Check sheet for the modelled part. Datum: model origin and axes. Units: mm. Face numbers are marked on the shaded views. A direction names the side the tool comes from. Round coordinates to 2 decimals unless told otherwise and drop trailing zeros. Write each loop counter-clockwise with the first axis right and the second up, starting at its lowest first coordinate (ties: lowest second). Pieces come first, ordered by that corner, then holes. Notation, with made-up numbers: M 50,50.5 L 67,50.5 A32 ccw 67,85.5 Z; hole C 29,73.25 d11. An arc over 180 degrees is marked long. Answer in a Markdown table with one row per item.
Autodesk Inventor part; units mm, degrees
ref_plane "YZ Plane" through (0, 0, 0) normal (1, 0, 0) x (0, 1, 0)
ref_plane "XZ Plane" through (0, 0, 0) normal (0, 1, 0) x (-1, 0, 0)
ref_plane "XY Plane" through (0, 0, 0) normal (0, 0, 1) x (1, 0, 0)
sketch "Sketch1" plane through (0, 0, 0) normal (0, 0, 1) x (1, 0, 0)
  line L0 (0, 0) -> (-122.2022, 0)
  line L1 (-122.2022, 0) -> (-122.2022, -1490)
  line L2 (-122.2022, -1490) -> (0, -1490)
  line L3 (0, -1490) -> (0, 0)
  line L4 (-122.2022, -1390) -> (-66, -1390)
  line L5 (-66, -1390) -> (-66, -1385)
  line L6 (-66, -1385) -> (-122.2022, -1385)
  line L7 (-122.2022, -1385) -> (-122.2022, -1390)
  line L8 (-122.2022, -893.3333) -> (-66, -893.3333)
  line L9 (-66, -893.3333) -> (-66, -888.3333)
  line L10 (-66, -888.3333) -> (-122.2022, -888.3333)
  line L11 (-122.2022, -888.3333) -> (-122.2022, -893.3333)
  line L12 (-122.2022, -396.6667) -> (-66, -396.6667)
  line L13 (-66, -396.6667) -> (-66, -391.6667)
  line L14 (-66, -391.6667) -> (-122.2022, -391.6667)
  line L15 (-122.2022, -391.6667) -> (-122.2022, -396.6667)
  circle A0 centre (-122.2022, -155) radius 30
  point P0 (-122.2022, -1385)
  point P1 (-122.2022, -125)
  point P2 (-122.2022, -185)
  dimension "d0" = 1490
  dimension "d1" = 122.2022
  dimension "d2" = 5
  dimension "d4" = 100
  dimension "d7" = 496.6667
  dimension "d23" = 66
  dimension "d28" = 60
  dimension "d29" = 1335
extrude "Plate1" add sketch "Sketch1" along normal blind 4 contours L3 L2 L1 L4 L5 L6 L8 L9 L10 L12 L13 L14 A0 L0
sketch "Sketch2" plane through (4, 0, 0) normal (-1, 0, 0) x (0, -1, 0)
  line L0 (1490, 0) -> (0, 0)
  line L1 (0, 0) -> (0, 60)
  line L2 (0, 60) -> (1490, 60)
  line L3 (1490, 60) -> (1490, 0)
edge flange "Flange1" height 60 angle 90 thickness 4 bend radius 4 thickness toward (-1, 0, 0) relief tear relief width 4 relief depth 2 edges at (0, -745, 4) wall of the first edge with corners at (4, -1490, 0) (4, 0, 0) (4, 0, 60) (4, -1490, 60)
bend "Bend1"
corner "Corner1"
chamfer "Corner Chamfer1" distance 3 angle 45 6 edges at (-122.2022, -1390, 2) (-122.2022, -1385, 2) (-122.2022, -893.3333, 2) (-122.2022, -888.3333, 2) (-122.2022, -391.6667, 2) (-122.2022, -396.6667, 2)
equation "\"d0\" = Стрингер_длина"
equation "\"d1\" = стрингер_глубина_7"
equation "\"d2\" = паз_под_стрингер_толщина"
equation "\"d7\" = 0.333333 * Стрингер_длина"
equation "\"d23\" = паз_под_стрингер_глубина - Thickness"
equation "\"d28\" = 2 * радиус_выреза_под_сварку"
equation "\"d12\" = Thickness"
equation "\"d13\" = BendReliefWidth"
equation "\"d14\" = BendReliefDepth"
equation "\"d15\" = MinimumRemnant"
equation "\"d16\" = TransitionRadius"
equation "\"d17\" = ребро_усилителей"
equation "\"d19\" = BendRadius"
equation "\"d20\" = CornerReliefSize"
equation "\"d21\" = GapSize"
equation "\"d22\" = JacobiRadiusSize"
equation "\"BendRadius\" = Thickness"
equation "\"BendReliefWidth\" = Thickness"
equation "\"BendReliefDepth\" = 0.5 * Thickness"
equation "\"CornerReliefSize\" = 4 * Thickness"
equation "\"MinimumRemnant\" = 2 * Thickness"
equation "\"TransitionRadius\" = BendRadius"
equation "\"JacobiRadiusSize\" = BendRadius"
equation "\"GapSize\" = Thickness"
properties part number "0381 GBK stringer 7" material "Steel"
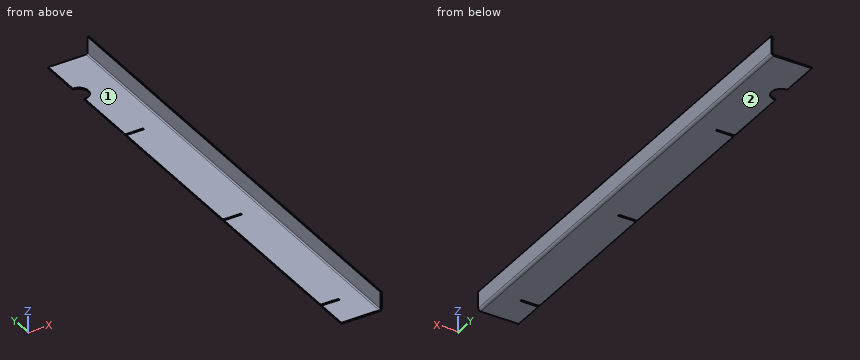
1. Section check D-D, the plane y = -333.5. Record the cut outline in (x, z).
Found:
| item | result |
|---|---|
| outline | M -122.2,0 L -4,0 A8 ccw 4,8 L 4,60 L 0,60 L 0,8 A4 cw -4,4 L -122.2,4 Z |
2. Section check A-A, the plane y = -155. Record the cut outline in (x, z), and give its area (3 significant figures).
Found:
| item | result |
|---|---|
| outline | M -92.2,0 L -4,0 A8 ccw 4,8 L 4,60 L 0,60 L 0,8 A4 cw -4,4 L -92.2,4 Z |
| area | 599 mm2 |
3. Access from +Z, -Z, +X, -X, +Y, -Y to the whole of each face (thin tool, end or side, straight path). Record for the marked faces 1 and 2.
Found:
| item | result |
|---|---|
| face 1 | +Z, -X, +Y, -Y |
| face 2 | -Z, +X, -X, +Y, -Y |
4. Go/stop test with flat-tipped pins: pin 1 (2 mm diameter, centred on y = -1387.5, z = 2, fed in from -X); pin 2 (6 mm diameter, centred on x = -11, y = -724, fed in from +Z); pin 3 (4.5 mm diameter, centred on y = -394.5, z = 2.5, fed in from -X). Record where each tip stops, or that it passes through.
Found:
| item | result |
|---|---|
| pin 1 | stops at x = -66 |
| pin 2 | stops at z = 4 |
| pin 3 | stops at x = -119.29 |
5. Section check C-C, the plane x = -39. Record the cut outline in (y, z).
Found:
| item | result |
|---|---|
| outline | M -1490,0 L 0,0 L 0,4 L -1490,4 Z |
6. Section check B-B, the plane z = 46.5. Record the cut outline in (x, y), and give its area (3 significant figures).
Found:
| item | result |
|---|---|
| outline | M 0,-1490 L 4,-1490 L 4,0 L 0,0 Z |
| area | 5,960 mm2 |
7. Scan lines: L1, parallel to Z at x = -71, y = -1404.5; L2, parallel to X at y = -407, z = 6. Record each from-to range of solid material in increasing order.
Found:
| item | result |
|---|---|
| L1 | z = 0 to 4 |
| L2 | x = -0.54 to 3.75 |
